For this review, take the finished solid that the model builds, in its own axes (mm). Give positions to 0.01 mm unless a question says otherwise; leave off trailing zeros. Write each loop counter-clockwise with the first axis right and the second up, starting at its lowest first coordinate (ties: lowest second). Pieces come first, ordered by that corner, then holes.
Q1. We need section D-D (y = 7.5). Give the number of separate pieces and of enclosed holes in the cut face, then the cut area to 3 significant figures.
Q2. We need section A-A (x = -300). Write out the cut boundary in (y, z), then the cut area to 3 significant figures.
Q3. We need section B-B (z = -45). Write out the cut boundary in (x, y), then the cut area to 3 significant figures.
Q4. For line 1 (X direction, y = 3.25, z = -250); line 2 (X direction, y = 9.75, z = -206); line 3 (X direction, y = 7, z = -220.85), list the stretches that pass through material, from the lowest coordinate up.
Q5. We need section C-C (x = -40). Write out the cut boundary in (y, z).
Q6. Insertion check: P1, Ø2, axis at y = 6, z = -50.5, coming from the +X side. The pin has a flat end and moves straight along its axis. Give the tip position at first contact, or say it passes through.
```python
from build123d import *

# Parameters (mm, degrees)
SCHIZZO1_W                   = 320
SCHIZZO1_H                   = 270
ESTRUSIONE_ESTRUSIONE1_DEPTH = 10
SCHIZZO3_R                   = 2.25
TAGLIO_ESTRUSIONE2_DEPTH     = 10
SCHIZZO4_R                   = 2.25
TAGLIO_ESTRUSIONE3_DEPTH     = 33
FORO_PER_VITE_M8_1_D         = 9
FORO_PER_VITE_M8_1_DEPTH     = 188
FORO_PER_VITE_M8_1_TIP       = 2.703872786
SCHIZZO7_R                   = 113
TAGLIO_ESTRUSIONE4_DEPTH     = 10
TAGLIO_ESTRUSIONE5_DEPTH     = 22
SCHIZZO9_R                   = 2.25
TAGLIO_ESTRUSIONE6_DEPTH     = 42.3
SCHIZZO10_W                  = 50.1
SCHIZZO10_H                  = 20.5
TAGLIO_ESTRUSIONE7_DEPTH     = 42.3
SCHIZZO11_R                  = 2.25
TAGLIO_ESTRUSIONE8_DEPTH     = 18
SCHIZZO12_R                  = 2.25
TAGLIO_ESTRUSIONE9_DEPTH     = 179
TAGLIO_ESTRUSIONE10_DEPTH    = 179


with BuildPart() as part:
    # Schizzo1 → Estrusione-Estrusione1 (new body)
    with BuildSketch(Plane(origin=(0, 0, 0), x_dir=(1, 0, 0), z_dir=(0, 1, 0))):
        with Locations((-160, 135)):
            Rectangle(SCHIZZO1_W, SCHIZZO1_H)
    extrude(amount=ESTRUSIONE_ESTRUSIONE1_DEPTH)

    # Schizzo3 → Taglio-Estrusione2 (cut)
    with BuildSketch(Plane(origin=(0, 10, 0), x_dir=(1, 0, 0), z_dir=(0, 1, 0))):
        with Locations(Location((-132.397041122, 205.611580849, 0), (0, 0, 270))):
            Circle(SCHIZZO3_R)
        with Locations(Location((-161.388419151, 155.397041122, 0), (0, 0, 270))):
            Circle(SCHIZZO3_R)
        with Locations(Location((-182.611580849, 234.602958878, 0), (0, 0, 270))):
            Circle(SCHIZZO3_R)
        with Locations(Location((-211.602958878, 184.388419151, 0), (0, 0, 270))):
            Circle(SCHIZZO3_R)
    extrude(amount=-TAGLIO_ESTRUSIONE2_DEPTH, mode=Mode.SUBTRACT)

    # Schizzo4 → Taglio-Estrusione3 (cut)
    with BuildSketch(Plane(origin=(0, 10, 0), x_dir=(1, 0, 0), z_dir=(0, 1, 0))):
        with Locations(Location((-272.0814314, 180.543373533, 0), (0, 0, 270))):
            Circle(SCHIZZO4_R)
        with Locations(Location((-249.710916031, 130.298373362, 0), (0, 0, 270))):
            Circle(SCHIZZO4_R)
        with Locations(Location((-94.289083758, 259.701626731, 0), (0, 0, 270))):
            Circle(SCHIZZO4_R)
        with Locations(Location((-71.918568389, 209.456626561, 0), (0, 0, 270))):
            Circle(SCHIZZO4_R)
        Polygon((-112.499215416, 236.816363994), (-104.785184586, 240.250871799), (-104.615474565, 246.89424924), (-77.861643306, 258.805822358), (-72.811093568, 254.486654307), (-65.097062738, 257.921162112), (-53.708436732, 232.341889298), (-61.422467562, 228.907381493), (-61.592177583, 222.264004053), (-88.346008842, 210.352430934), (-93.396558579, 214.671598985), (-101.110589409, 211.23709118), align=None)
        Polygon((-242.88941038, 178.762908913), (-231.500784374, 153.183636099), (-239.214815204, 149.749128294), (-239.384525224, 143.105750854), (-266.138356484, 131.194177735), (-271.188906221, 135.513345787), (-278.902937051, 132.078837982), (-290.291563058, 157.658110796), (-282.577532228, 161.092618601), (-282.407822207, 167.735996041), (-255.653990947, 179.64756916), (-250.60344121, 175.328401108), align=None)
    extrude(amount=-TAGLIO_ESTRUSIONE3_DEPTH, mode=Mode.SUBTRACT)

    # Foro per Vite M8-1
    with Locations(Plane(origin=(0, 10, 0), x_dir=(1, 0, 0), z_dir=(0, 1, 0))):
        with Locations((-300, 20), (-300, 250), (-40, 250), (-40, 20)):
            Hole(FORO_PER_VITE_M8_1_D / 2, depth=FORO_PER_VITE_M8_1_DEPTH)
            with Locations((0, 0, -(FORO_PER_VITE_M8_1_DEPTH + FORO_PER_VITE_M8_1_TIP / 2))):  # 118° drill point
                Cone(0, FORO_PER_VITE_M8_1_D / 2, FORO_PER_VITE_M8_1_TIP, mode=Mode.SUBTRACT)

    # Schizzo7 → Taglio-Estrusione4 (cut)
    with BuildSketch(Plane(origin=(0, 10, 0), x_dir=(1, 0, 0), z_dir=(0, 1, 0))):
        with Locations((33, 140)):
            Circle(SCHIZZO7_R)
    extrude(amount=-TAGLIO_ESTRUSIONE4_DEPTH, mode=Mode.SUBTRACT)

    # Schizzo8 → Taglio-Estrusione5 (cut)
    with BuildSketch(Plane(origin=(0, 10, 0), x_dir=(1, 0, 0), z_dir=(0, 1, 0))):
        Polygon((-280.401232083, 238), (-276.401232083, 242), (-242.101232083, 242), (-238.101232083, 238), (-238.101232083, 203.7), (-242.101232083, 199.7), (-276.401232083, 199.7), (-280.401232083, 203.7), align=None)
    extrude(amount=-TAGLIO_ESTRUSIONE5_DEPTH, mode=Mode.SUBTRACT)

    # Schizzo9 → Taglio-Estrusione6 (cut)
    with BuildSketch(Plane(origin=(0, 10, 0), x_dir=(1, 0, 0), z_dir=(0, 1, 0))):
        with Locations(Location((-228.601232, 220.85, 0), (0, 0, 270))):
            Circle(SCHIZZO9_R)
        with Locations(Location((-289.901232, 220.85, 0), (0, 0, 270))):
            Circle(SCHIZZO9_R)
    extrude(amount=-TAGLIO_ESTRUSIONE6_DEPTH, mode=Mode.SUBTRACT)

    # Schizzo10 → Taglio-Estrusione7 (cut)
    with BuildSketch(Plane(origin=(0, 10, 0), x_dir=(1, 0, 0), z_dir=(0, 1, 0))):
        with Locations((-177.95, 109)):
            Rectangle(SCHIZZO10_W, SCHIZZO10_H)
    extrude(amount=-TAGLIO_ESTRUSIONE7_DEPTH, mode=Mode.SUBTRACT)

    # Schizzo11 → Taglio-Estrusione8 (cut)
    with BuildSketch(Plane(origin=(0, 10, 0), x_dir=(1, 0, 0), z_dir=(0, 1, 0))):
        with Locations(Location((-182, 91.25, 0), (0, 0, 270))):
            Circle(SCHIZZO11_R)
        with Locations(Location((-182, 126.75, 0), (0, 0, 270))):
            Circle(SCHIZZO11_R)
    extrude(amount=-TAGLIO_ESTRUSIONE8_DEPTH, mode=Mode.SUBTRACT)

    # Schizzo12 → Taglio-Estrusione9 (cut)
    with BuildSketch(Plane(origin=(0, 10, 0), x_dir=(1, 0, 0), z_dir=(0, 1, 0))):
        with Locations(Location((-95.652024181, 202.266681741, 0), (0, 0, 270))):
            Circle(SCHIZZO12_R)
        with Locations(Location((-130.721715924, 130.363158037, 0), (0, 0, 270))):
            Circle(SCHIZZO12_R)
    extrude(amount=-TAGLIO_ESTRUSIONE9_DEPTH, mode=Mode.SUBTRACT)

    # Schizzo13 → Taglio-Estrusione10 (cut)
    with BuildSketch(Plane(origin=(0, 10, 0), x_dir=(1, 0, 0), z_dir=(0, 1, 0))):
        with BuildLine():
            Line((-191.594117082, 52.5), (-156.594117082, 52.5))
            ThreePointArc((-156.594117082, 52.5), (-149.094117082, 45), (-156.594117082, 37.5))
            Line((-156.594117082, 37.5), (-191.594117082, 37.5))
            ThreePointArc((-191.594117082, 37.5), (-199.094117082, 45), (-191.594117082, 52.5))
        make_face()
    extrude(amount=-TAGLIO_ESTRUSIONE10_DEPTH, mode=Mode.SUBTRACT)


solid = part.part
```
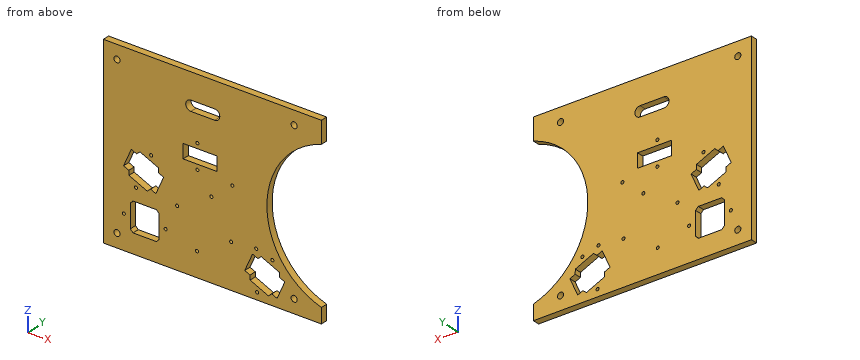
Computed:
1. separate pieces: 1
1. enclosed holes: 23
1. area: 66,100 mm2
2. outline: (0, -270) - (10, -270) - (10, -254.5) - (0, -254.5) - close; (0, -245.5) - (10, -245.5) - (10, -24.5) - (0, -24.5) - close; (0, -15.5) - (10, -15.5) - (10, 0) - (0, 0) - close
2. area: 2,520 mm2
3. outline: (-320, 0) - (-199.09, 0) - (-199.09, 10) - (-320, 10) - close; (-149.09, 0) - (-28.19, 0) - (-28.19, 10) - (-149.09, 10) - close
3. area: 2,420 mm2
4. line 1: x = -320 to -304.5, -295.5 to -97.64, -61.57 to -44.5, -35.5 to 0
4. line 2: x = -320 to -280.4, -238.1 to -134.61, -130.18 to -58.72
4. line 3: x = -320 to -292.15, -287.65 to -280.4, -238.1 to -230.85, -226.35 to -105.39, -64.77 to -45.94
5. outline: (0, -270) - (10, -270) - (10, -254.5) - (0, -254.5) - close; (0, -245.5) - (10, -245.5) - (10, -226.26) - (0, -226.26) - close; (0, -53.74) - (10, -53.74) - (10, -24.5) - (0, -24.5) - close; (0, -15.5) - (10, -15.5) - (10, 0) - (0, 0) - close
6. P1: stops at x = -34.67
